```python
from build123d import *

# Parameters (mm, degrees)
BOSS_EXTRUDE1_DEPTH = 10
SKETCH2_W           = 20.36
SKETCH2_H           = 8
BOSS_EXTRUDE2_DEPTH = 30
BOSS_EXTRUDE3_DEPTH = 10
SKETCH4_R           = 1.8
CUT_EXTRUDE1_DEPTH  = 90.301874976
CUT_EXTRUDE2_DEPTH  = 90.301874976
FILLET2_R           = 10
FILLET3_R           = 2
FILLET4_R           = 2
SKETCH6_W           = 9
SKETCH6_H           = 20
CUT_EXTRUDE3_DEPTH  = 5
SKETCH7_W           = 9
SKETCH7_H           = 20
CUT_EXTRUDE4_DEPTH  = 5
SKETCH8_W           = 10
SKETCH8_H           = 63.5
BOSS_EXTRUDE4_DEPTH = 4.5
SKETCH9_W           = 10
SKETCH9_H           = 5
BOSS_EXTRUDE5_DEPTH = 15
SKETCH10_W          = 10
SKETCH10_H          = 63.5
BOSS_EXTRUDE6_DEPTH = 4.5
SKETCH11_W          = 10
SKETCH11_H          = 5
BOSS_EXTRUDE7_DEPTH = 15
SKETCH12_R          = 1.8
CUT_EXTRUDE5_DEPTH  = 5


with BuildPart() as part:
    # Sketch1 → Boss-Extrude1 (new body)
    with BuildSketch(Plane.XY):
        Polygon((-68.691883613, -39.730446699), (-48.331883613, -39.730446699), (-48.331883613, -14.230446699), (10.268116387, -14.230446699), (10.268116387, -39.730446699), (30.628116387, -39.730446699), (30.628116387, -4.230446699), (-68.691883613, -4.230446699), align=None)
    extrude(amount=BOSS_EXTRUDE1_DEPTH)

    # Sketch2 → Boss-Extrude2 (add)
    with BuildSketch(Plane.XY.offset(10)):
        with Locations((-58.511883613, -35.730446699)):
            Rectangle(SKETCH2_W, SKETCH2_H)
        with Locations((20.448116387, -35.730446699)):
            Rectangle(SKETCH2_W, SKETCH2_H)
    extrude(amount=BOSS_EXTRUDE2_DEPTH)

    # Sketch3 → Boss-Extrude3 (add)
    with BuildSketch(Plane.XY.offset(40)):
        Polygon((-68.691883613, -39.730446699), (-68.691883613, -4.230446699), (30.628116387, -4.230446699), (30.628116387, -39.730446699), (10.268116387, -39.730446699), (10.268116387, -14.230446699), (-48.331883613, -14.230446699), (-48.331883613, -39.730446699), align=None)
    extrude(amount=BOSS_EXTRUDE3_DEPTH)

    # Sketch4 → Cut-Extrude1 (cut, through all)
    with BuildSketch(Plane(origin=(0, -31.730446699, 0), x_dir=(1, 0, 0), z_dir=(0, 1, 0))):
        with Locations(Location((-58.511883613, -20, 0), (0, 0, 270))):
            Circle(SKETCH4_R)
        with Locations(Location((-58.511883613, -30, 0), (0, 0, 270))):
            Circle(SKETCH4_R)
        with Locations(Location((20.448116387, -30, 0), (0, 0, 270))):
            Circle(SKETCH4_R)
        with Locations(Location((20.448116387, -20, 0), (0, 0, 270))):
            Circle(SKETCH4_R)
    extrude(amount=-CUT_EXTRUDE1_DEPTH, mode=Mode.SUBTRACT)

    # Sketch5 → Cut-Extrude2 (cut, through all)
    with BuildSketch(Plane(origin=(0, -31.730446699, 0), x_dir=(1, 0, 0), z_dir=(0, 1, 0))):
        with BuildLine():
            Line((-68.691883613, -13.5), (-65.691883613, -13.5))
            ThreePointArc((-65.691883613, -13.5), (-64.277670051, -14.085786438), (-63.691883613, -15.5))
            Line((-63.691883613, -15.5), (-63.691883613, -34.5))
            ThreePointArc((-63.691883613, -34.5), (-64.277670051, -35.914213562), (-65.691883613, -36.5))
            Line((-65.691883613, -36.5), (-68.691883613, -36.5))
            Line((-68.691883613, -36.5), (-68.691883613, -13.5))
        make_face()
        with BuildLine():
            Line((30.628116387, -13.174954518), (27.628116387, -13.174954518))
            ThreePointArc((27.628116387, -13.174954518), (26.213902825, -13.760740955), (25.628116387, -15.174954518))
            Line((25.628116387, -15.174954518), (25.628116387, -34.174954518))
            ThreePointArc((25.628116387, -34.174954518), (26.213902825, -35.58916808), (27.628116387, -36.174954518))
            Line((27.628116387, -36.174954518), (30.628116387, -36.174954518))
            Line((30.628116387, -36.174954518), (30.628116387, -13.174954518))
        make_face()
    extrude(amount=-CUT_EXTRUDE2_DEPTH, mode=Mode.SUBTRACT)

    # Fillet2
    fillet2_edges = [part.edges().sort_by_distance(p)[0] for p in [
        (30.628116387, -4.230446699, 5),
        (30.628116387, -4.230446699, 45),
        (-68.691883613, -4.230446699, 5),
        (-68.691883613, -4.230446699, 45),
    ]]
    fillet(fillet2_edges, radius=FILLET2_R)

    # Fillet3
    fillet3_edges = [part.edges().sort_by_distance(p)[0] for p in [
        (20.448116387, -31.730446699, 40),
        (-58.511883613, -31.730446699, 40),
        (20.448116387, -31.730446699, 10),
        (-58.511883613, -31.730446699, 10),
    ]]
    fillet(fillet3_edges, radius=FILLET3_R)

    # Fillet4
    fillet4_edges = [part.edges().sort_by_distance(p)[0] for p in [
        (10.268116387, -21.980446699, 10),
        (-48.331883613, -21.980446699, 40),
        (10.268116387, -31.730446699, 25),
        (-48.331883613, -31.730446699, 25),
        (-48.331883613, -21.980446699, 10),
        (10.268116387, -31.144660261, 39.414213562),
        (-48.331883613, -31.144660261, 39.414213562),
        (10.268116387, -31.144660261, 10.585786438),
        (-48.331883613, -31.144660261, 10.585786438),
        (10.268116387, -21.980446699, 40),
    ]]
    fillet(fillet4_edges, radius=FILLET4_R)

    # Sketch6 → Cut-Extrude3 (cut)
    with BuildSketch(Plane.XY.offset(50)):
        with Locations((-58.511883613, -29.730446699)):
            Rectangle(SKETCH6_W, SKETCH6_H)
        with Locations((20.448116387, -29.730446699)):
            Rectangle(SKETCH6_W, SKETCH6_H)
    extrude(amount=-CUT_EXTRUDE3_DEPTH, mode=Mode.SUBTRACT)

    # Sketch7 → Cut-Extrude4 (cut)
    with BuildSketch(Plane(origin=(0, 0, 0), x_dir=(-1, 0, 0), z_dir=(0, 0, -1))):
        with Locations((-20.448116387, -29.730446699)):
            Rectangle(SKETCH7_W, SKETCH7_H)
        with Locations((58.511883613, -29.730446699)):
            Rectangle(SKETCH7_W, SKETCH7_H)
    extrude(amount=-CUT_EXTRUDE4_DEPTH, mode=Mode.SUBTRACT)

    # Sketch8 → Boss-Extrude4 (add)
    with BuildSketch(Plane(origin=(30.628116387, 0, 0), x_dir=(0, 0, -1), z_dir=(1, 0, 0))):
        with Locations((-45, -7.980446699)):
            Rectangle(SKETCH8_W, SKETCH8_H)
        with Locations((-5, -7.980446699)):
            Rectangle(SKETCH8_W, SKETCH8_H)
    extrude(amount=BOSS_EXTRUDE4_DEPTH)

    # Sketch9 → Boss-Extrude5 (add)
    with BuildSketch(Plane.ZY.offset(-30.628116387)):
        with Locations((5, 21.269553301)):
            Rectangle(SKETCH9_W, SKETCH9_H)
        with Locations((45, 21.269553301)):
            Rectangle(SKETCH9_W, SKETCH9_H)
    extrude(amount=BOSS_EXTRUDE5_DEPTH)

    # Sketch10 → Boss-Extrude6 (add)
    with BuildSketch(Plane.ZY.offset(68.691883613)):
        with Locations((5, -7.980446699)):
            Rectangle(SKETCH10_W, SKETCH10_H)
        with Locations((45, -7.980446699)):
            Rectangle(SKETCH10_W, SKETCH10_H)
    extrude(amount=BOSS_EXTRUDE6_DEPTH)

    # Sketch11 → Boss-Extrude7 (add)
    with BuildSketch(Plane(origin=(-68.691883613, 0, 0), x_dir=(0, 0, -1), z_dir=(1, 0, 0))):
        with Locations((-45, 21.269553301)):
            Rectangle(SKETCH11_W, SKETCH11_H)
        with Locations((-5, 21.269553301)):
            Rectangle(SKETCH11_W, SKETCH11_H)
    extrude(amount=BOSS_EXTRUDE7_DEPTH)

    # Sketch12 → Cut-Extrude5 (cut)
    with BuildSketch(Plane(origin=(0, 23.769553301, 0), x_dir=(1, 0, 0), z_dir=(0, 1, 0))):
        with Locations(Location((20.448116387, -45, 0), (0, 0, 270))):
            Circle(SKETCH12_R)
        with Locations(Location((20.448116387, -5, 0), (0, 0, 270))):
            Circle(SKETCH12_R)
        with Locations(Location((-58.511883613, -45, 0), (0, 0, 270))):
            Circle(SKETCH12_R)
        with Locations(Location((-58.511883613, -5, 0), (0, 0, 270))):
            Circle(SKETCH12_R)
    extrude(amount=-CUT_EXTRUDE5_DEPTH, mode=Mode.SUBTRACT)


solid = part.part
```
Here's how the part is built. I have some questions about the finished solid (model axes, mm). A direction names the side the tool comes from. Coordinates: 2 decimals unless noted, no trailing zeros. Loops run counter-clockwise (first coordinate to the right, second up) from the corner with the lowest first, then second, coordinate; pieces in that order, holes last. Notation, with made-up numbers: (-3, 67) -> (32, 67) arc R8 cw to (32, 82) -> close; hole circle Ø1 at (75.25, 12). An arc over 180 degrees is marked (long way). Return JSON: item names as keys, results as strings.
1) For faces 1 (the face through (29, -36, 13.175)), 2 (the face through (-56.727, 21.305, 44.766)), 3 (the face through (-58, -30, 5)), 4 (the face through (-59, -30, 45)), which set-ups out of +Z, -Z, +X, -X, +Y, -Y let a thin tool reach every point of the face, with its end or its side?
Results below:
{"face 1": "+X, +Y, -Y", "face 2": "+Y", "face 3": "-Z, -Y", "face 4": "+Z, -Y"}
2) If we section it at D-D, the plane y = -9: Write out the boundary of the cut face in (x, z).
Results below:
{"outline": "(-73.19, 0) -> (-68.69, 0) -> (-68.69, 10) -> (-73.19, 10) -> close; (-73.19, 40) -> (-68.69, 40) -> (-68.69, 50) -> (-73.19, 50) -> close; (-67.21, 0) -> (29.15, 0) -> (29.15, 10) -> (-67.21, 10) -> close; (-67.21, 40) -> (29.15, 40) -> (29.15, 50) -> (-67.21, 50) -> close; (30.63, 0) -> (35.13, 0) -> (35.13, 10) -> (30.63, 10) -> close; (30.63, 40) -> (35.13, 40) -> (35.13, 50) -> (30.63, 50) -> close"}
3) Will these pins go through, and if not, where does the flat tip stop? pin 1 (12 mm diameter, centred on x = 20.5, z = 27, fed in from +Y); pin 2 (3 mm diameter, centred on x = 20.45, z = 20, fed in from -Y); pin 3 (2.5 mm diameter, centred on y = -34.5, z = 27, fed in from +X); pin 4 (2 mm diameter, centred on x = -32, z = 6, fed in from -Y).
Results below:
{"pin 1": "y = -31.73", "pin 2": "through", "pin 3": "x = 25.63", "pin 4": "y = -14.23"}
4) Thinking about a two-plate mould opening in X: for faces 5 (the face through (30.628, -36, 38)), 6 (the face through (-63, 23.77, 5)), 7 (the face through (-68.692, 3, 5)), which applies, +X half, -X half, draft (parallel to the pull), parting line (faces both ways), or undercut?
Results below:
{"face 5": "+X half", "face 6": "draft", "face 7": "undercut"}
5) If we section it at A-A, the plane z = 30: Write out the boundary of the cut face in (x, y), then the cut area to 3 significant figures.
Results below:
{"outline": "(-63.69, -39.73) -> (-60.31, -39.73) -> (-60.31, -31.73) -> (-63.69, -31.73) -> close; (-56.71, -39.73) -> (-48.33, -39.73) -> (-48.33, -33.73) arc R2 ccw to (-50.33, -31.73) -> (-56.71, -31.73) -> close; (10.27, -39.73) -> (18.65, -39.73) -> (18.65, -31.73) -> (12.27, -31.73) arc R2 ccw to (10.27, -33.73) -> close; (22.25, -39.73) -> (25.63, -39.73) -> (25.63, -31.73) -> (22.25, -31.73) -> close", "area": "186 mm²"}
6) If we section it at C-C, the plane x = 6: Write out the boundary of the cut face in (y, z), then the cut area to 3 significant figures.
Results below:
{"outline": "(-14.23, 0) -> (-4.23, 0) -> (-4.23, 10) -> (-14.23, 10) -> close; (-14.23, 40) -> (-4.23, 40) -> (-4.23, 50) -> (-14.23, 50) -> close", "area": "200 mm²"}
7) I need wall thicknesses on line 1 (X direction, y = -36, z = 30); line 2 (X direction, y = 20.75, z = 5); line 3 (Z direction, x = -63.5, y = -6). Which ranges of each line are inside material? Lowest first, please. Write a range as from..to.
Results below:
{"line 1": "-63.69..-60.31, -56.71..-48.33, 10.27..18.65, 22.25..25.63", "line 2": "-73.19..-60.31, -56.71..-53.69, 15.63..18.65, 22.25..35.13", "line 3": "0..10, 40..50"}
8) If we section it at B-B, the plane y = 2: Write out the boundary of the cut face in (x, z), then the cut area to 3 significant figures.
Results below:
{"outline": "(-73.19, 0) -> (-68.69, 0) -> (-68.69, 10) -> (-73.19, 10) -> close; (-73.19, 40) -> (-68.69, 40) -> (-68.69, 50) -> (-73.19, 50) -> close; (30.63, 0) -> (35.13, 0) -> (35.13, 10) -> (30.63, 10) -> close; (30.63, 40) -> (35.13, 40) -> (35.13, 50) -> (30.63, 50) -> close", "area": "180 mm²"}
